Design review of the part built by this model. Coordinates are the model's own, in mm. Face numbers are marked on the shaded views. A direction names the side the tool comes from. Coordinates: 2 decimals unless noted, no trailing zeros. Loops run counter-clockwise (first coordinate to the right, second up) from the corner with the lowest first, then second, coordinate; pieces in that order, holes last. Notation, with made-up numbers: M 82,-39.75 L 104,-39.75 A18 cw 104,-10.75 Z; hole C 88.25,87 d3. An arc over 180 degrees is marked long. One line per item, written item: value.
```python
from build123d import *

# Parameters (mm, degrees)
F0_W     = 127
F0_H     = 101.6
F1_DEPTH = 19.05
F2_T     = -2.54
F3_R     = 3.175
F4_DEPTH = 2.54
F5_R     = 4.7625
F6_DEPTH = 2.54


with BuildPart() as f1:
    # F0 (on Front) → F1 (new body, symmetric)
    with BuildSketch(Plane.XZ):
        Rectangle(F0_W, F0_H)
    extrude(amount=F1_DEPTH, both=True)

    # F2
    f2_openings = [f1.faces().sort_by_distance(p)[0] for p in [
        (0, 19.05, 0),
    ]]
    offset(amount=F2_T, openings=f2_openings)

    # F3 (on face) → F4 (cut, through all)
    with BuildSketch(Plane.YZ.offset(63.5)):
        with Locations((0, -38.1)):
            Circle(F3_R)
        with Locations((0, 12.7)):
            Circle(F3_R)
    extrude(amount=-F4_DEPTH, mode=Mode.SUBTRACT)

    # F5 (on face) → F6 (cut, through all)
    with BuildSketch(Plane(origin=(-63.5, 0, 0), x_dir=(0, -1, 0), z_dir=(-1, 0, 0))):
        with Locations((0, 38.1)):
            Circle(F5_R)
        Circle(F5_R)
    extrude(amount=-F6_DEPTH, mode=Mode.SUBTRACT)


solid = f1.part
```
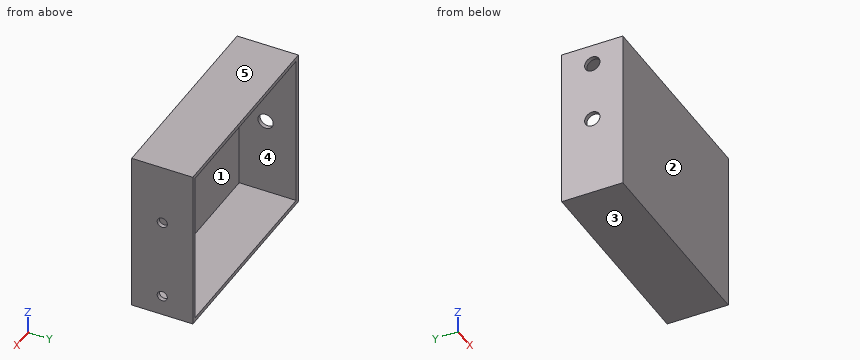
(1) We need section C-C on y = 0. State the section outline as (x, z) points (1 decimal), then the cut area to 3 significant figures.
Reply:
outline: M -63.5,-50.8 L 63.5,-50.8 L 63.5,-41.3 L 61,-41.3 L 61,-48.3 L -61,-48.3 L -61,-4.8 L -63.5,-4.8 Z; M -63.5,4.8 L -61,4.8 L -61,33.3 L -63.5,33.3 Z; M -63.5,42.9 L -61,42.9 L -61,48.3 L 61,48.3 L 61,15.9 L 63.5,15.9 L 63.5,50.8 L -63.5,50.8 Z; M 61,-34.9 L 63.5,-34.9 L 63.5,9.5 L 61,9.5 Z
area: 1,050 mm2
(2) Tool access review of the marked faces 1 and 2: name each direction out of +Z, -Z, +X, -X, +Y, -Y from which nothing blocks a thin tool from reaching the whole face with its end or side.
Reply:
face 1: +Y
face 2: +Z, -Z, +X, -X, -Y
(3) Mouldability with a two-part tool opening along Z and no side actions: class the marked faces 3, 4 and 5 as released by +Z, released by -Z, zero draft, split by the parting line, or undercut.
Reply:
face 3: released by -Z
face 4: undercut
face 5: released by +Z
(4) We need section A-A on z = 12.7. State the section outline as (x, y) points (3 decimals).
Reply:
outline: M -63.5,-19.05 L 63.5,-19.05 L 63.5,-3.175 L 60.96,-3.175 L 60.96,-16.51 L -60.96,-16.51 L -60.96,19.05 L -63.5,19.05 Z; M 60.96,3.175 L 63.5,3.175 L 63.5,19.05 L 60.96,19.05 Z
(5) To check wall thickness, follow line 1 along Z through (x, y) = (-62.5, 0); line 2 along Z through (x, y) = (62.1, 0) (3 decimals); line 3 along X through (y, z) = (-10.5, -41). State the ranges of each line that lie inside material, in increasing order. Write a range as [from, to].
Reply:
line 1: z = [-50.8, -4.76], [4.76, 33.34], [42.86, 50.8]
line 2: z = [-50.8, -41.275], [-34.925, 9.525], [15.875, 50.8]
line 3: x = [-63.5, -60.96], [60.96, 63.5]
(6) We need section B-B on y = 16. State the section outline as (x, z) points, then the cut area to 3 significant figures.
Reply:
outline: M -63.5,-50.8 L 63.5,-50.8 L 63.5,50.8 L -63.5,50.8 Z; hole M -60.96,-48.26 L 60.96,-48.26 L 60.96,48.26 L -60.96,48.26 Z
area: 1,140 mm2
(7) We need section D-D on x = 55. State the section outline as (y, z) points.
Reply:
outline: M -19.05,-50.8 L 19.05,-50.8 L 19.05,-48.26 L -16.51,-48.26 L -16.51,48.26 L 19.05,48.26 L 19.05,50.8 L -19.05,50.8 Z
